Part model, mm, in its own coordinate system. A direction names the side the tool comes from. Give positions to 0.01 mm unless a question says otherwise; leave off trailing zeros. Write each loop counter-clockwise with the first axis right and the second up, starting at its lowest first coordinate (ties: lowest second). Pieces come first, ordered by that corner, then holes. Notation, with made-up numbers: M -28,3 L 15,3 A19 cw 15,9 Z; hole C 46.5,79 d3. An arc over 180 degrees is marked long. Answer as CSV lines item,"result". Start each with the question number.
Item 1: Wall check: L1, parallel to Z at x = 33, y = 0.35; L2, parallel to X at y = 1.5, z = -69; L3, parallel to X at y = 3.4, z = -55 (3 decimals). Give the ranges that are in metal, low to high. Write a range as from..to.
Item 2: Band-saw the part on B-B, the plane z = -62. List the corners of the cut face in (x, y) (3 decimals).
Item 3: Band-saw the part on C-C, the plane y = 0.9. Count the separate pieces of the cut face and the enclosed holes in it, then the cut area to 3 significant figures.
Item 4: Band-saw the part on D-D, the plane x = 43.5. List the corners of the cut face in (y, z).
Item 5: Pin check, flat tips, straight feed: pin 1 (1 mm diameter, centred on x = 27.5, y = 2, fed in from +Z); pin 2 (1.7 mm diameter, centred on y = 3, z = -60.5, fed in from -X) (3 decimals); pin 3 (1 mm diameter, centred on x = 19, y = 4.5, fed in from +Z). Stop position of each tip, or through.
Item 6: Band-saw the part on A-A, the plane x = 1. List the corners of the cut face in (y, z).
Item 7: 3-axis set-ups, long thin cutter, end or side, ignore diameter. For faces 4 (the flat face through (18, 3, -66.701)), 5 (the flat face through (56.765, 3, -58)), 6 (the cylindrical face through (31.724, 2.755, -66.661)): which of +Z, -Z, +X, -X, +Y, -Y reach the whole face in a straight line?
Item 8: Two-plate mould, pull along Z, no slides. Class faces 1 (the flat face through (48, 3, -66.701)), 2 (the cylindrical face through (67.88, 2.75, -5.5)), 3 (the flat face through (32, 0, -32)): +Z half, -Z half, draft (parallel to the pull), parting line (faces both ways), or undercut.
from build123d import *

# Parameters (mm, degrees)
SKETCH1_R                  = 35
SKETCH1_R_2                = 6
SKETCH1_R_3                = 5
SKETCH1_R_4                = 2.3
SKETCH1_W                  = 47.96
SKETCH1_H                  = 25
BOSS_EXTRUDE3_DEPTH        = 5.588
F_4_6_4_6_DIAMETER_HOLE1_D = 4.6
FILLET1_R                  = 3
FILLET2_R                  = 2
FILLET3_R                  = 2
FILLET4_R                  = 1


with BuildPart() as part:
    # Sketch1 → Boss-Extrude3 (new body)
    # profile 1 of 5: a face of its own
    with BuildSketch(Plane(origin=(0, 0, 0), x_dir=(1, 0, 0), z_dir=(0, 1, 0))):
        with Locations((32.785, 23.351471482)):
            Circle(SKETCH1_R)
        with Locations(Location((32.785, 23.351471482, 0), (0, 0, 270))):
            Circle(SKETCH1_R_2, mode=Mode.SUBTRACT)
    # profile 2 of 5: a face of its own
    with BuildSketch(Plane(origin=(0, 0, 0), x_dir=(1, 0, 0), z_dir=(0, 1, 0))):
        with Locations((65.600049901, 5.201471482)):
            Circle(SKETCH1_R_3)
        with Locations(Location((65.600049901, 5.201471482, 0), (0, 0, 270))):
            Circle(SKETCH1_R_4, mode=Mode.SUBTRACT)
    # profile 3 of 5: a face of its own
    with BuildSketch(Plane(origin=(0, 0, 0), x_dir=(1, 0, 0), z_dir=(0, 1, 0))):
        with Locations((-0.030049901, 5.201471482)):
            Circle(SKETCH1_R_3)
        with Locations(Location((-0.030049901, 5.201471482, 0), (0, 0, 270))):
            Circle(SKETCH1_R_4, mode=Mode.SUBTRACT)
    # profile 4 of 5: a face of its own
    with BuildSketch(Plane(origin=(0, 0, 0), x_dir=(1, 0, 0), z_dir=(0, 1, 0))):
        with Locations((32.785, 68.701471482)):
            Circle(SKETCH1_R_3)
    # profile 5 of 5: a face of its own
    with BuildSketch(Plane(origin=(0, 0, 0), x_dir=(1, 0, 0), z_dir=(0, 1, 0))):
        with Locations((32.785, 54.201471482)):
            Rectangle(SKETCH1_W, SKETCH1_H)
    extrude(amount=BOSS_EXTRUDE3_DEPTH)

    # Ø4.6 (4.6) Diameter Hole1 (through all)
    with Locations(Plane(origin=(0, 5.588, 0), x_dir=(1, 0, 0), z_dir=(0, 1, 0))):
        with Locations((32.785, 68.701471482)):
            Hole(F_4_6_4_6_DIAMETER_HOLE1_D / 2)

    # Fillet1
    fillet1_edges = [part.edges().sort_by_distance(p)[0] for p in [
        (65.214711372, 2.794, -10.18660079),
        (61.172514444, 2.794, -2.878342174),
        (0.355288628, 2.794, -10.18660079),
        (4.397485556, 2.794, -2.878342174),
    ]]
    fillet(fillet1_edges, radius=FILLET1_R)

    # Fillet2
    fillet2_edges = [part.edges().sort_by_distance(p)[0] for p in [
        (28.202424305, 2.794, -66.701471482),
        (37.367575695, 2.794, -66.701471482),
    ]]
    fillet(fillet2_edges, radius=FILLET2_R)

    # Fillet3
    fillet3_edges = [part.edges().sort_by_distance(p)[0] for p in [
        (8.805, 2.794, -48.845776728),
        (56.765, 2.794, -48.845776728),
    ]]
    fillet(fillet3_edges, radius=FILLET3_R)

    # Fillet4
    fillet4_edges = [part.edges().sort_by_distance(p)[0] for p in [
        (56.765, 2.794, -66.701471482),
        (8.805, 2.794, -66.701471482),
    ]]
    fillet(fillet4_edges, radius=FILLET4_R)


solid = part.part
Output:
1,L1,"-73.7..-70.99, -66.41..-29.35, -17.36..11.65"
1,L2,"27.79..30.5, 35.07..37.78"
1,L3,"8.805..56.765"
2,outline,"M 8.805,0 L 56.765,0 L 56.765,5.588 L 8.805,5.588 Z"
3,separate pieces,"1"
3,enclosed holes,"4"
3,area,"4,430 mm²"
4,outline,"M 0,-66.7 L 5.59,-66.7 L 5.59,9.97 L 0,9.97 Z"
5,pin 1,"z = 11.32"
5,pin 2,"x = 8.805"
5,pin 3,"z = 9.03"
6,outline,"M 0,-38 L 5.59,-38 L 5.59,-7.26 L 0,-7.26 Z; M 0,-3.15 L 5.59,-3.15 L 5.59,-0.31 L 0,-0.31 Z"
7,face 4,"-Z, -X, +Y, -Y"
7,face 5,"-Z, +X, +Y, -Y"
7,face 6,"+Y, -Y"
8,face 1,"-Z half"
8,face 2,"undercut"
8,face 3,"draft"
